from build123d import *

# Parameters (mm, degrees)
SKETCH1_W                                      = 139.7
SKETCH1_H                                      = 127
BOSS_EXTRUDE1_DEPTH                            = 6.35
CUT_EXTRUDE1_DEPTH                             = 7.35
F_4_40_TAPPED_HOLE1_D                          = 2.2606
F_4_40_TAPPED_HOLE1_DEPTH                      = 7.5946
F_4_40_TAPPED_HOLE1_TIP                        = 0.679152758
F_4_40_TAPPED_HOLE2_D                          = 2.2606
F_4_40_TAPPED_HOLE2_DEPTH                      = 7.5946
F_4_40_TAPPED_HOLE2_TIP                        = 0.679152758
F_4_40_TAPPED_HOLE3_D                          = 2.2606
F_4_40_TAPPED_HOLE3_DEPTH                      = 7.5946
F_4_40_TAPPED_HOLE3_TIP                        = 0.679152758
CBORE_FOR_4_SOCKET_HEAD_CAP_SCREW1_D           = 3.2639
CBORE_FOR_4_SOCKET_HEAD_CAP_SCREW1_DEPTH       = 7.5946
CBORE_FOR_4_SOCKET_HEAD_CAP_SCREW1_CBORE_D     = 5.55752
CBORE_FOR_4_SOCKET_HEAD_CAP_SCREW1_CBORE_DEPTH = 2.8448
CBORE_FOR_4_SOCKET_HEAD_CAP_SCREW1_TIP         = 0.980574487
F_4_40_TAPPED_HOLE4_D                          = 2.2606
F_4_40_TAPPED_HOLE4_DEPTH                      = 7.5946
F_4_40_TAPPED_HOLE4_TIP                        = 0.679152758
FILLET1_R                                      = 3.175


with BuildPart() as part:
    # Sketch1 → Boss-Extrude1 (new body)
    with BuildSketch(Plane.XY):
        Rectangle(SKETCH1_W, SKETCH1_H)
    extrude(amount=BOSS_EXTRUDE1_DEPTH)

    # Sketch2 → Cut-Extrude1 (cut, through all)
    with BuildSketch(Plane.XY.offset(6.35)):
        Polygon((-57.15, 50.8), (-57.15, -50.8), (-12.7, 0), align=None)
        Polygon((57.15, 50.8), (57.15, -50.8), (12.7, 0), align=None)
        Polygon((-31.75, 50.8), (31.75, 50.8), (0, 14.514285714), align=None)
        Polygon((31.75, -50.8), (0, -14.514285714), (-31.75, -50.8), align=None)
    extrude(amount=-CUT_EXTRUDE1_DEPTH, mode=Mode.SUBTRACT)

    # #4-40 Tapped Hole1
    with Locations(Plane(origin=(0, -63.5, 0), x_dir=(-1, 0, 0), z_dir=(0, -1, 0))):
        with Locations((-63.5, -3.175), (63.5, -3.175)):
            Hole(F_4_40_TAPPED_HOLE1_D / 2, depth=F_4_40_TAPPED_HOLE1_DEPTH)
            with Locations((0, 0, -(F_4_40_TAPPED_HOLE1_DEPTH + F_4_40_TAPPED_HOLE1_TIP / 2))):  # 118° drill point
                Cone(0, F_4_40_TAPPED_HOLE1_D / 2, F_4_40_TAPPED_HOLE1_TIP, mode=Mode.SUBTRACT)

    # #4-40 Tapped Hole2
    with Locations(Plane.ZY.offset(69.85)):
        with Locations((3.175, 0), (3.175, 50.8), (3.175, -50.8)):
            Hole(F_4_40_TAPPED_HOLE2_D / 2, depth=F_4_40_TAPPED_HOLE2_DEPTH)
            with Locations((0, 0, -(F_4_40_TAPPED_HOLE2_DEPTH + F_4_40_TAPPED_HOLE2_TIP / 2))):  # 118° drill point
                Cone(0, F_4_40_TAPPED_HOLE2_D / 2, F_4_40_TAPPED_HOLE2_TIP, mode=Mode.SUBTRACT)

    # #4-40 Tapped Hole3
    with Locations(Plane(origin=(69.85, 0, 0), x_dir=(0, 0, -1), z_dir=(1, 0, 0))):
        with Locations((-3.175, 50.8), (-3.175, 0), (-3.175, -50.8)):
            Hole(F_4_40_TAPPED_HOLE3_D / 2, depth=F_4_40_TAPPED_HOLE3_DEPTH)
            with Locations((0, 0, -(F_4_40_TAPPED_HOLE3_DEPTH + F_4_40_TAPPED_HOLE3_TIP / 2))):  # 118° drill point
                Cone(0, F_4_40_TAPPED_HOLE3_D / 2, F_4_40_TAPPED_HOLE3_TIP, mode=Mode.SUBTRACT)

    # CBORE for #4 Socket Head Cap Screw1
    with Locations(Plane(origin=(0, 0, 0), x_dir=(-1, 0, 0), z_dir=(0, 0, -1))):
        with Locations((0, 0)):
            CounterBoreHole(CBORE_FOR_4_SOCKET_HEAD_CAP_SCREW1_D / 2, CBORE_FOR_4_SOCKET_HEAD_CAP_SCREW1_CBORE_D / 2, CBORE_FOR_4_SOCKET_HEAD_CAP_SCREW1_CBORE_DEPTH, depth=CBORE_FOR_4_SOCKET_HEAD_CAP_SCREW1_DEPTH)
            with Locations((0, 0, -(CBORE_FOR_4_SOCKET_HEAD_CAP_SCREW1_DEPTH + CBORE_FOR_4_SOCKET_HEAD_CAP_SCREW1_TIP / 2))):  # 118° drill point
                Cone(0, CBORE_FOR_4_SOCKET_HEAD_CAP_SCREW1_D / 2, CBORE_FOR_4_SOCKET_HEAD_CAP_SCREW1_TIP, mode=Mode.SUBTRACT)

    # #4-40 Tapped Hole4
    with Locations(Plane(origin=(0, 63.5, 0), x_dir=(1, 0, 0), z_dir=(0, 1, 0))):
        with Locations((-63.5, -3.175), (63.5, -3.175)):
            Hole(F_4_40_TAPPED_HOLE4_D / 2, depth=F_4_40_TAPPED_HOLE4_DEPTH)
            with Locations((0, 0, -(F_4_40_TAPPED_HOLE4_DEPTH + F_4_40_TAPPED_HOLE4_TIP / 2))):  # 118° drill point
                Cone(0, F_4_40_TAPPED_HOLE4_D / 2, F_4_40_TAPPED_HOLE4_TIP, mode=Mode.SUBTRACT)

    # Fillet1
    fillet1_edges = [part.edges().sort_by_distance(p)[0] for p in [
        (0, 14.514285714, 3.175),
        (-31.75, 50.8, 3.175),
        (31.75, 50.8, 3.175),
        (31.75, -50.8, 3.175),
        (-31.75, -50.8, 3.175),
        (0, -14.514285714, 3.175),
        (12.7, 0, 3.175),
        (57.15, 50.8, 3.175),
        (57.15, -50.8, 3.175),
        (-57.15, 50.8, 3.175),
        (-12.7, 0, 3.175),
        (-57.15, -50.8, 3.175),
    ]]
    fillet(fillet1_edges, radius=FILLET1_R)


solid = part.part
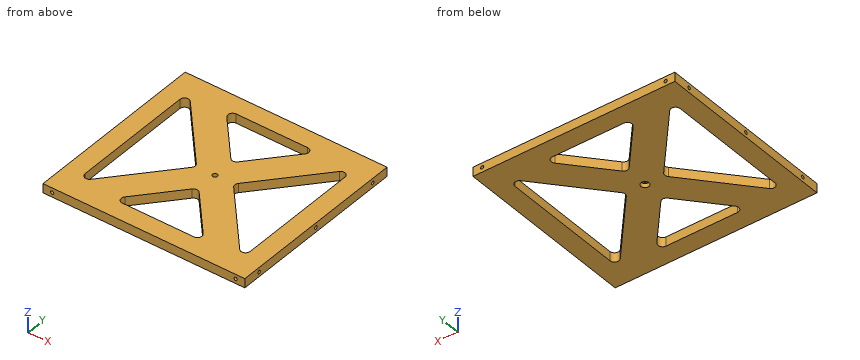
Geometry check sheet. Reference: the model listing, model coordinates, mm. Give positions to 0.01 mm unless a question says otherwise; leave off trailing zeros. Loops run counter-clockwise (first coordinate to the right, second up) from the corner with the lowest first, then second, coordinate; pieces in that order, holes last.
(1) Thickness scan on L1, parallel to X at y = 6.5, z = 3.5; L2, parallel to Z at x = -64.75, y = 0; L3, parallel to Y at x = -54, z = 6.25. Record the ranges inside material, lowest first.
From the geometry:
L1: x = -69.85 to -57.15, -18.39 to 18.39, 57.15 to 69.85
L2: z = 0 to 2.04, 4.31 to 6.35
L3: y = -63.5 to -45.52, 45.52 to 63.5
(2) Section check B-B on y = 12. Record the cut outline in (x, z), then the cut area to 3 significant figures.
From the geometry:
outline: (-69.85, 0) - (-57.15, 0) - (-57.15, 6.35) - (-69.85, 6.35) - close; (-23.2, 0) - (23.2, 0) - (23.2, 6.35) - (-23.2, 6.35) - close; (57.15, 0) - (69.85, 0) - (69.85, 6.35) - (57.15, 6.35) - close
area: 456 mm2
(3) Section check C-C on z = 1. Count the separate pieces of the cut face and the enclosed holes in it, then the cut area to 3 significant figures.
From the geometry:
separate pieces: 1
enclosed holes: 5
area: 11,000 mm2
(4) Depth check by flat-ended pin: pin 1 Ø1.8 at (y, z) = (50.8, 3.175) entering from -X; pin 2 Ø2 at (y, z) = (-50.8, 3.175) entering from -X; pin 3 Ø2 at (x, y) = (0, 0) entering from -Z; pin 4 Ø1.8 at (x, z) = (-63.5, 3.175) entering from +Y. Enter the tip coordinate at first touch or a pass-through.
From the geometry:
pin 1: stops at x = -62.12
pin 2: stops at x = -62.18
pin 3: passes through
pin 4: stops at y = 55.77
(5) Section check D-D on x = 36.5. Record the cut outline in (y, z), then the cut area to 3 significant figures.
From the geometry:
outline: (-63.5, 0) - (-27.2, 0) - (-27.2, 6.35) - (-63.5, 6.35) - close; (27.2, 0) - (63.5, 0) - (63.5, 6.35) - (27.2, 6.35) - close
area: 461 mm2
(6) Section check A-A on x = 0. Record the cut outline in (y, z).
From the geometry:
outline: (-63.5, 0) - (-50.8, 0) - (-50.8, 6.35) - (-63.5, 6.35) - close; (-16.16, 0) - (-2.78, 0) - (-2.78, 2.84) - (-1.63, 2.84) - (-1.63, 6.35) - (-16.16, 6.35) - close; (1.63, 2.84) - (2.78, 2.84) - (2.78, 0) - (16.16, 0) - (16.16, 6.35) - (1.63, 6.35) - close; (50.8, 0) - (63.5, 0) - (63.5, 6.35) - (50.8, 6.35) - close
